Check sheet for the drawn part. Datum: minimum x, y, z corner. Units: mm. Coordinates: 2 decimals unless noted, no trailing zeros. Loops run counter-clockwise (first coordinate to the right, second up) from the corner with the lowest first, then second, coordinate; pieces in that order, holes last.
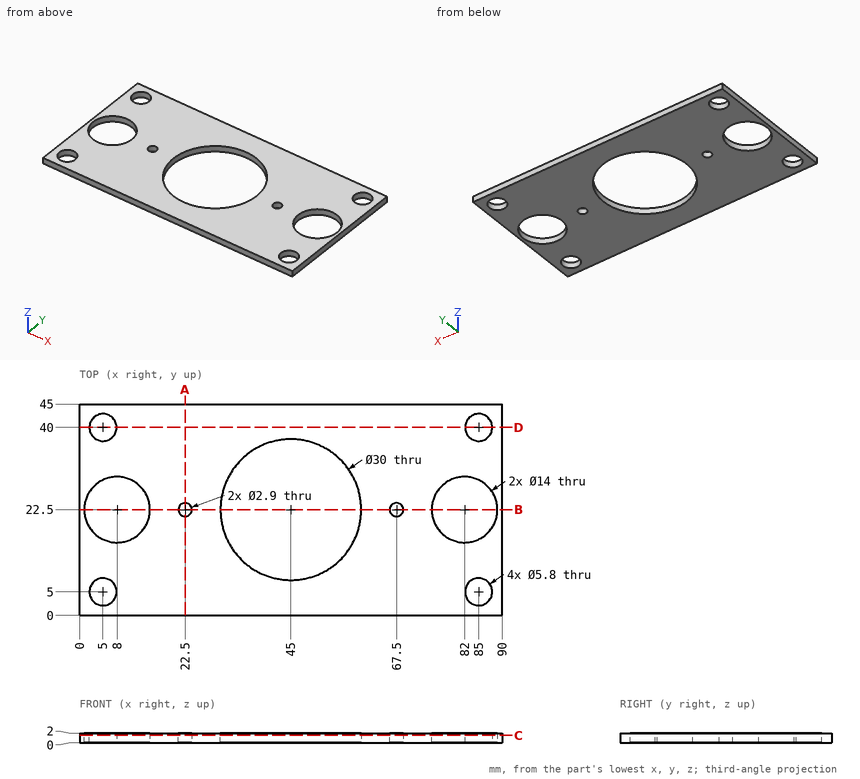
(1) Scan lines: L1, parallel to Y at x = 45, z = 0.7; L2, parallel to X at y = 38, z = 1.15; L3, parallel to X at y = 19, z = 1.45. Record each from-to range of solid material in increasing order.
Findings:
L1: y = 0 to 7.5, 37.5 to 45
L2: x = 0 to 2.9, 7.1 to 82.9, 87.1 to 90
L3: x = 0 to 1.94, 14.06 to 30.41, 59.59 to 75.94, 88.06 to 90
(2) Sectioned sample at C-C on z = 1.55. State how many separate pieces and enclosed holes the cut face has, and give its area (3 significant figures).
Findings:
separate pieces: 1
enclosed holes: 9
area: 2,920 mm2
(3) Sectioned sample at A-A on x = 22.5. Record the cut outline in (y, z), and give its area (3 significant figures).
Findings:
outline: (0, 0) - (21.05, 0) - (21.05, 2) - (0, 2) - close; (23.95, 0) - (45, 0) - (45, 2) - (23.95, 2) - close
area: 84.2 mm2
(4) Sectioned sample at D-D on y = 40. Record the cut outline in (x, z), and give its area (3 significant figures).
Findings:
outline: (0, 0) - (2.1, 0) - (2.1, 2) - (0, 2) - close; (7.9, 0) - (82.1, 0) - (82.1, 2) - (7.9, 2) - close; (87.9, 0) - (90, 0) - (90, 2) - (87.9, 2) - close
area: 157 mm2
(5) Sectioned sample at B-B on y = 22.5. Record the cut outline in (x, z).
Findings:
outline: (0, 0) - (1, 0) - (1, 2) - (0, 2) - close; (15, 0) - (21.05, 0) - (21.05, 2) - (15, 2) - close; (23.95, 0) - (30, 0) - (30, 2) - (23.95, 2) - close; (60, 0) - (66.05, 0) - (66.05, 2) - (60, 2) - close; (68.95, 0) - (75, 0) - (75, 2) - (68.95, 2) - close; (89, 0) - (90, 0) - (90, 2) - (89, 2) - close
(6) Gauge pin test, flat end, axial feed: pin 1 Ø3.5 at (x, y) = (5, 5) entering from -Z. Record the tip position at first contact, or that the pin passes through.
Findings:
pin 1: passes through
